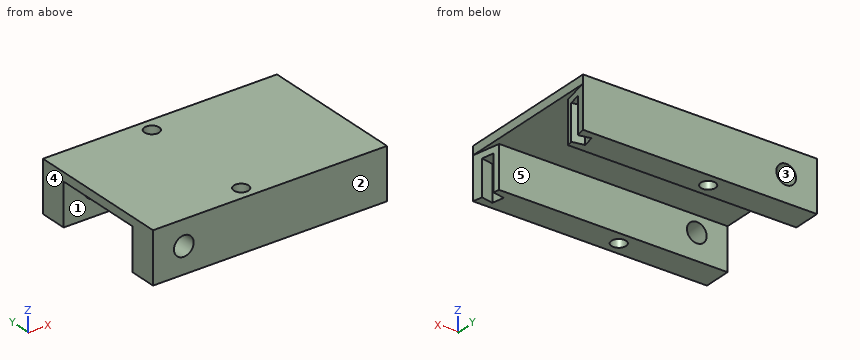
from build123d import *

# Parameters (mm, degrees)
SKETCH1_W           = 15
SKETCH1_H           = 4.12
BOSS_EXTRUDE1_DEPTH = 12
SKETCH3_W           = 3.42
SKETCH3_H           = 7.5
CUT_EXTRUDE1_DEPTH  = 25
CUT_EXTRUDE3_DEPTH  = 3.42
SKETCH7_W           = 2.9
SKETCH7_H           = 1
CUT_EXTRUDE4_DEPTH  = 1
BOSS_EXTRUDE2_DEPTH = 4


with BuildPart() as part:
    # Sketch1 → Boss-Extrude1 (new body)
    with BuildSketch(Plane(origin=(0, 0, 0), x_dir=(1, 0, 0), z_dir=(0, 1, 0))):
        with Locations((7.5, 2.06)):
            Rectangle(SKETCH1_W, SKETCH1_H)
    extrude(amount=BOSS_EXTRUDE1_DEPTH)

    # Sketch3 → Cut-Extrude1 (cut)
    with BuildSketch(Plane.ZY):
        with Locations((-2.41, 6)):
            Rectangle(SKETCH3_W, SKETCH3_H)
    extrude(amount=-CUT_EXTRUDE1_DEPTH, mode=Mode.SUBTRACT)

    # Sketch5 → Cut-Extrude3 (cut)
    with BuildSketch(Plane(origin=(0, 0, -4.12), x_dir=(-1, 0, 0), z_dir=(0, 0, -1))):
        Polygon((-15, 12), (-14.55, 9.75), (-15, 9.75), align=None)
    cut_extrude3 = extrude(amount=-CUT_EXTRUDE3_DEPTH, mode=Mode.SUBTRACT)

    # Mirror2: Cut-Extrude3 across plane
    add(cut_extrude3.mirror(Plane(origin=(0, 6, 0), x_dir=(0, 0, 1), z_dir=(0, -1, 0))), mode=Mode.SUBTRACT)

    # Sketch7 → Cut-Extrude4 (cut)
    with BuildSketch(Plane(origin=(12.115384617, -2.423076922, 0), x_dir=(0, 0, -1), z_dir=(0.9805806757046813, -0.19611613506937897, 0))):
        with Locations((2.67, 13.414151353)):
            Rectangle(SKETCH7_W, SKETCH7_H)
    cut_extrude4 = extrude(amount=-CUT_EXTRUDE4_DEPTH, mode=Mode.SUBTRACT)

    # Sketch10 → #0-80 Tapped Hole1 (revolve, cut)
    with BuildSketch(Plane(origin=(4, 10.875, -4.12), x_dir=(0, 1, 0), z_dir=(1, 0, 0))):
        Polygon((0, 0), (0, 5.307890611), (0.59563, 4.95), (0.59563, 0), align=None)
    f_0_80_tapped_hole1 = revolve(axis=Axis((4, 10.875, -10.47), (0, 0, 1)), mode=Mode.SUBTRACT)

    # Sketch12 → Boss-Extrude2 (add)
    with BuildSketch(Plane.ZY):
        Polygon((0, 0), (0, 12), (-4.12, 12), (-4.12, 9.75), (-0.7, 9.75), (-0.7, 2.25), (-4.12, 2.25), (-4.12, 0), align=None)
    extrude(amount=BOSS_EXTRUDE2_DEPTH)

    # Sketch15 → M2x0.4 Tapped Hole1 (revolve, cut)
    with BuildSketch(Plane(origin=(-1.5, 12, -2), x_dir=(0, 0, 1), z_dir=(1, 0, 0))):
        Polygon((0, 0), (0, 5.680688495), (0.8, 5.2), (0.8, 0), align=None)
    m2x0_4_tapped_hole1 = revolve(axis=Axis((-1.5, 18.35, -2), (0, -1, 0)), mode=Mode.SUBTRACT)

    # Mirror3: Cut-Extrude4, #0-80 Tapped Hole1, M2x0.4 Tapped Hole1 across plane
    add(cut_extrude4.mirror(Plane(origin=(0, 6, 0), x_dir=(0, 0, 1), z_dir=(0, -1, 0))), mode=Mode.SUBTRACT)
    add(f_0_80_tapped_hole1.mirror(Plane(origin=(0, 6, 0), x_dir=(0, 0, 1), z_dir=(0, -1, 0))), mode=Mode.SUBTRACT)
    add(m2x0_4_tapped_hole1.mirror(Plane(origin=(0, 6, 0), x_dir=(0, 0, 1), z_dir=(0, -1, 0))), mode=Mode.SUBTRACT)


solid = part.part
CAD build for the part. Positions are in the model's coordinates, mm. Face numbers are marked on the shaded views. A direction names the side the tool comes from. Round coordinates to 2 decimals unless told otherwise and drop trailing zeros. Loops run counter-clockwise (first coordinate to the right, second up) from the corner with the lowest first, then second, coordinate; pieces in that order, holes last.
(1) Wall check: line 1 along Y through (x, z) = (4, -1.7); line 2 along Y through (x, z) = (1, -0.9); line 3 along Z through (x, y) = (-1.5, 1.6). Give the ranges that are in metal, low to high.
(2) Cut at C-C (x = 4). Give the cut face in (y, z), plus the area to 3 significant figures.
(3) Which spindle directions (+Z, -Z, +X, -X, +Y, -Y) get a long thin tool onto all of the face, cutting with end or side? Do the marked faces 4 and 5. Say none if no direction does.
(4) Cut at D-D (x = 11.75). Give the cut face in (y, z).
(5) Cut at B-B (z = -0.9). Give the cut face in (x, y) (3 decimals), plus the area to 3 significant figures.
(6) Two-plate mould, pull along Y, no slides. Class the marked faces 1, 2 and 3: +Y half, -Y half, draft (parallel to the pull), parting line (faces both ways), or undercut.
(7) Cut at A-A (z = -2). Give the cut face in (x, y) (3 decimals).
Findings below:
1. line 1: y = 0 to 0.53, 1.72 to 2.25, 9.75 to 10.28, 11.47 to 12
1. line 2: y = 0 to 2.25, 9.75 to 12
1. line 3: z = -4.12 to -2.8, -1.2 to 0
2. outline: (0, -4.12) - (0.53, -4.12) - (0.53, 0) - (0, 0) - close; (1.72, -4.12) - (2.25, -4.12) - (2.25, -0.7) - (9.75, -0.7) - (9.75, -4.12) - (10.28, -4.12) - (10.28, 0) - (1.72, 0) - close; (11.47, -4.12) - (12, -4.12) - (12, 0) - (11.47, 0) - close
2. area: 14.0 mm2
3. face 4: +Z, -Z, -X, +Y, -Y
3. face 5: -Z, +X, -X
4. outline: (0, -4.12) - (2.25, -4.12) - (2.25, -0.7) - (9.75, -0.7) - (9.75, -4.12) - (12, -4.12) - (12, 0) - (0, 0) - close
5. outline: (-4, 0) - (15, 0) - (14.55, 2.25) - (-4, 2.25) - close; (-4, 9.75) - (14.55, 9.75) - (15, 12) - (-4, 12) - close; hole circle Ø1.191 at (4, 1.125); hole circle Ø1.191 at (4, 10.875)
5. area: 82.3 mm2
6. face 1: undercut
6. face 2: -Y half
6. face 3: draft
7. outline: (-4, 0) - (-2.3, 0) - (-2.3, 2.25) - (-4, 2.25) - close; (-4, 9.75) - (-2.3, 9.75) - (-2.3, 12) - (-4, 12) - close; (-0.7, 0) - (15, 0) - (14.844, 0.779) - (13.864, 0.583) - (13.667, 1.564) - (14.648, 1.76) - (14.55, 2.25) - (-0.7, 2.25) - close; (-0.7, 9.75) - (14.55, 9.75) - (14.648, 10.24) - (13.667, 10.436) - (13.864, 11.417) - (14.844, 11.221) - (15, 12) - (-0.7, 12) - close; hole circle Ø1.191 at (4, 1.125); hole circle Ø1.191 at (4, 10.875)
